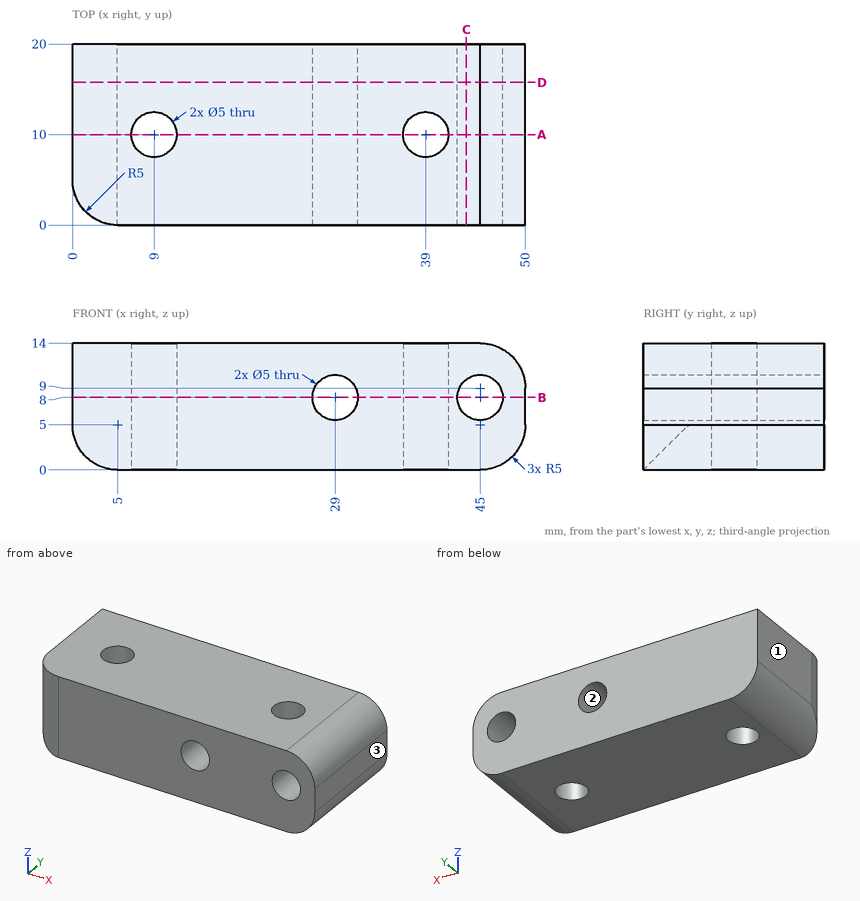
Design review of the part shown in the three views and the two pictorial views. Dimensions are in mm from the part's minimum x, y and z. Round coordinates to 2 decimals unless told otherwise and drop trailing zeros. Write each loop counter-clockwise with the first axis right and the second up, starting at its lowest first coordinate (ties: lowest second). Pieces come first, ordered by that corner, then holes. Notation, with made-up numbers: M -20,75 L 6,75 A18 cw 6,106 Z; hole C 4,70 d10. An arc over 180 degrees is marked long. Use a Markdown table: item, result. Add a question column.
Q1. Insertion check: pin 1 (6 mm diameter, centred on x = 39, y = 10, fed in from +Z); pin 2 (4 mm diameter, centred on x = 45, z = 8, fed in from +Y). Each pin has a flat end and moves straight along its axis. Give the tip position at first contact, or say it passes through.
Q2. We need section D-D, the plane y = 15.75. State the section outline as (x, z) points, plus the area to 3 significant figures.
Q3. The part is to be moulded in two halves that separate along X. For the marked faces 1, 2 and 3, say which applies: pulls with the +X half, pulls with the -X half, needs draft (parallel to the pull), parting line crosses it, or undercut.
Q4. We need section B-B, the plane z = 8. State the section outline as (x, y) points.
Q5. We need section A-A, the plane y = 10. State the section outline as (x, z) points, plus the area to 3 significant figures.
Q6. We need section C-C, the plane x = 43.5. State the section outline as (y, z) points, plus the area to 3 significant figures.
Q7. To check wall thickness, follow line 1 (Y direction, x = 9, z = 10.5); line 2 (Z direction, x = 29, y = 13); line 3 (X direction, y = 10.5, z = 2.25). State the ranges of each line that lie inside material, in increasing order.
Findings below:
| question | item | result |
|---|---|---|
| 1 | pin 1 | stops at z = 14 |
| 1 | pin 2 | passes through |
| 2 | outline | M 0,4.97 A5 ccw 4.97,0 L 45.03,0 A5 ccw 50,4.97 L 50,9.03 A5 ccw 45.03,14 L 0,14 Z; hole C 29,8 d5; hole C 45,8 d5 |
| 2 | area | 645 mm² |
| 3 | face 1 | pulls with the -X half |
| 3 | face 2 | undercut |
| 3 | face 3 | pulls with the +X half |
| 4 | outline | M 0,5 A5 ccw 5,0 L 26.5,0 L 26.5,20 L 0,20 Z; M 31.5,0 L 42.5,0 L 42.5,20 L 31.5,20 Z; M 47.5,0 L 50,0 L 50,20 L 47.5,20 Z; hole C 9,10 d5; hole C 39,10 d5 |
| 5 | outline | M 0,4.97 A5 ccw 4.97,0 L 6.5,0 L 6.5,14 L 0,14 Z; M 11.5,0 L 36.5,0 L 36.5,14 L 11.5,14 Z; M 41.5,0 L 45.03,0 A5 ccw 50,4.97 L 50,9.03 A5 ccw 45.03,14 L 41.5,14 Z; hole C 29,8 d5; hole C 45,8 d5 |
| 5 | area | 505 mm² |
| 6 | outline | M 0,0 L 20,0 L 20,6 L 0,6 Z; M 0,10 L 20,10 L 20,14 L 0,14 Z |
| 6 | area | 200 mm² |
| 7 | line 1 | y = 0 to 7.5, 12.5 to 20 |
| 7 | line 2 | z = 0 to 5.5, 10.5 to 14 |
| 7 | line 3 | x = 0.82 to 6.55, 11.45 to 36.55, 41.45 to 49.18 |
